Here's how the part is built. I have some questions about the finished solid (model axes, mm). A direction names the side the tool comes from. Round coordinates to 2 decimals unless told otherwise and drop trailing zeros. Write each loop counter-clockwise with the first axis right and the second up, starting at its lowest first coordinate (ties: lowest second). Pieces come first, ordered by that corner, then holes. Notation, with made-up numbers: (19.5, -32) -> (77.5, -32) arc R17 ccw to (77.5, -13) -> close; hole circle Ø7 at (39.25, 54.5). An arc over 180 degrees is marked (long way). Put each result on its own line as item: value. Start each with the question number.
1. I need wall thicknesses on probe 1 along X at (y, z) = (6.75, 0.5); probe 2 along Z at (x, y) = (-24.5, -1.5); probe 3 along Y at (x, z) = (-43.5, 2). Which ranges of each line are inside material? Lowest first, please. Write a range as from..to.
2. For pin 1 (10 mm diameter, centred on y = -8, z = -5, fed in from -X); pin 2 (4.5 mm diameter, centred on y = -3, z = -0.5, fed in from +X); pin 3 (4 mm diameter, centred on x = 27.5, z = 42.5, fed in from +Y); pin 4 (3 mm diameter, centred on x = 0.5, y = -4.5, fed in from +Z), each with a flat end and sliding along its axis, tell me the tip position at first contact or that it passes through.
3. Suppose I cut it at C-C (z = 0). Count the separate pieces of the cut face and the enclosed holes in it, then the cut area to 3 significant figures.
4. We'd pull the mould along X, two halves only. Please class faces 4 (the face through (0.515, 6.479, -49.897)), 5 (the face through (29.846, 4.93, 31.091)), 6 (the face through (26, -3, -10)): +X half, -X half, draft (parallel to the pull), parting line (faces both ways), or undercut.
5. Suppose I cut it at A-A (y = -2). Please give me the cut outline in (x, z).
6. Suppose I cut it at B-B (y = -10). Please give me the cut outline in (x, z), then the cut area to 3 significant figures.
7. Which directions (+Z, -Z, +X, -X, +Y, -Y) give clear straight access to the entire face, cutting with the end or side of a thin tool? Please do faces 1 (the face through (0, -5, 15)), 2 (the face through (21.71, -0.99, -2.53)), 3 (the face through (-28, 3.5, 3.2)).
```python
from build123d import *
from OCP.BRepFilletAPI import BRepFilletAPI_MakeChamfer

# Parameters (mm, degrees)
SKETCH_1_R          = 55
EXTRUDE_1_DEPTH     = 5
SKETCH_2_R          = 49.9
EXTRUDE_2_DEPTH     = 5
SKETCH_3_W          = 35
SKETCH_3_H          = 30
EXTRUDE_3_DEPTH     = 25
SKETCH_4_W          = 20.2
SKETCH_4_H          = 10.3
CUT_EXTRUDE_1_DEPTH = 93.466210045
SKETCH_5_R          = 4.1
CUT_EXTRUDE_2_DEPTH = 82.700673192
SKETCH_6_R          = 2.75
CUT_EXTRUDE_3_DEPTH = 86.293610546
CHAMFER1_SIZE       = 2
CHAMFER1_SIZE2      = 0.535898385
SKETCH2_W           = 35
SKETCH2_H           = 30
CUT_EXTRUDE1_DEPTH  = 12.5
BOSS_EXTRUDE1_START = -2
SKETCH4_W           = 70
SKETCH4_H           = 20
BOSS_EXTRUDE1_DEPTH = 5.35
SKETCH5_R           = 4.15
CUT_EXTRUDE2_DEPTH  = 80.281917882
CUT_EXTRUDE3_DEPTH  = 6.5
SKETCH7_W           = 20
SKETCH7_H           = 34
CUT_EXTRUDE4_DEPTH  = 5
CHAMFER2_SIZE       = 1
CHAMFER2_SIZE2      = 2.747477419


with BuildPart() as part:
    # Эскиз1 → Бобышка-Вытянуть1 (new body)
    with BuildSketch(Plane(origin=(0, 0, 0), x_dir=(1, 0, 0), z_dir=(0, 1, 0))):
        with Locations(Location((0, 0, 0), (0, 0, 270))):
            Circle(SKETCH_1_R)
    extrude(amount=EXTRUDE_1_DEPTH)

    # Эскиз2 → Бобышка-Вытянуть2 (add)
    with BuildSketch(Plane(origin=(0, 5, 0), x_dir=(1, 0, 0), z_dir=(0, 1, 0))):
        with Locations(Location((0, 0, 0), (0, 0, 270))):
            Circle(SKETCH_2_R)
    extrude(amount=EXTRUDE_2_DEPTH)

    # Эскиз3 → Бобышка-Вытянуть3 (add)
    with BuildSketch(Plane.XZ):
        Rectangle(SKETCH_3_W, SKETCH_3_H)
    extrude(amount=EXTRUDE_3_DEPTH)

    # Эскиз4 → Вырез-Вытянуть1 (cut, through all)
    with BuildSketch(Plane.XY.offset(15)):
        with Locations((0, -12.5)):
            Rectangle(SKETCH_4_W, SKETCH_4_H)
    extrude(amount=-CUT_EXTRUDE_1_DEPTH, mode=Mode.SUBTRACT)

    # Эскиз5 → Вырез-Вытянуть2 (cut, through all)
    with BuildSketch(Plane.XZ):
        with Locations(Location((33.592198598, -32.871936263, 0), (0, 0, 270))):
            Circle(SKETCH_5_R)
        with Locations(Location((-33.591727056, -32.872418125, 0), (0, 0, 270))):
            Circle(SKETCH_5_R)
        with Locations(Location((-33.591727056, 32.872418125, 0), (0, 0, 270))):
            Circle(SKETCH_5_R)
        with Locations(Location((33.483215177, 32.983215177, 0), (0, 0, 270))):
            Circle(SKETCH_5_R)
    extrude(amount=-CUT_EXTRUDE_2_DEPTH, mode=Mode.SUBTRACT)

    # Эскиз6 → Вырез-Вытянуть3 (cut, through all)
    with BuildSketch(Plane(origin=(0, 10, 0), x_dir=(1, 0, 0), z_dir=(0, 1, 0))):
        with Locations(Location((-17.999856554, 19.999999999, 0), (0, 0, 270))):
            Circle(SKETCH_6_R)
    extrude(amount=-CUT_EXTRUDE_3_DEPTH, mode=Mode.SUBTRACT)

    # Chamfer1: one chamfer whose edges measure the first distance from different faces: ONE call of the kernel's chamfer builder (chamfer() names one face for all edges)
    chamfer1_edges_1 = [part.edges().sort_by_distance(p)[0] for p in [
        (0.000357897, 10, -49.899999999),
    ]]
    chamfer1_side_1 = [part.faces().sort_by_distance(p)[0] for p in [
        (0.000357897, 7.5, -49.899999999),
    ]]
    chamfer1_edges_2 = [part.edges().sort_by_distance(p)[0] for p in [
        (-49.9, 10, 0),
    ]]
    chamfer1_side_2 = [part.faces().sort_by_distance(p)[0] for p in [
        (-49.9, 7.5, 0),
    ]]
    chamfer1_edges_3 = [part.edges().sort_by_distance(p)[0] for p in [
        (-0.08242255, 10, 49.899931929),
    ]]
    chamfer1_side_3 = [part.faces().sort_by_distance(p)[0] for p in [
        (-0.08242255, 7.5, 49.899931929),
    ]]
    chamfer1_edges_4 = [part.edges().sort_by_distance(p)[0] for p in [
        (49.899931657, 10, 0.082587101),
    ]]
    chamfer1_side_4 = [part.faces().sort_by_distance(p)[0] for p in [
        (49.899931657, 7.5, 0.082587101),
    ]]
    chamfer1 = BRepFilletAPI_MakeChamfer(part.part.solid().wrapped)
    for e in chamfer1_edges_1:
        chamfer1.Add(CHAMFER1_SIZE, CHAMFER1_SIZE2, e.wrapped, chamfer1_side_1[0].wrapped)  # the first distance lies on this face
    for e in chamfer1_edges_2:
        chamfer1.Add(CHAMFER1_SIZE, CHAMFER1_SIZE2, e.wrapped, chamfer1_side_2[0].wrapped)  # the first distance lies on this face
    for e in chamfer1_edges_3:
        chamfer1.Add(CHAMFER1_SIZE, CHAMFER1_SIZE2, e.wrapped, chamfer1_side_3[0].wrapped)  # the first distance lies on this face
    for e in chamfer1_edges_4:
        chamfer1.Add(CHAMFER1_SIZE, CHAMFER1_SIZE2, e.wrapped, chamfer1_side_4[0].wrapped)  # the first distance lies on this face
    add(Compound.cast(chamfer1.Shape()), mode=Mode.REPLACE)

    # Sketch2 → Cut-Extrude1 (cut)
    with BuildSketch(Plane.XZ.offset(25)):
        Rectangle(SKETCH2_W, SKETCH2_H)
    extrude(amount=-CUT_EXTRUDE1_DEPTH, mode=Mode.SUBTRACT)

    # Sketch4 → Boss-Extrude1 (add)
    with BuildSketch(Plane.XZ.offset(7.35).offset(BOSS_EXTRUDE1_START)):
        Rectangle(SKETCH4_W, SKETCH4_H)
    extrude(amount=-BOSS_EXTRUDE1_DEPTH)

    # Sketch5 → Cut-Extrude2 (cut, through all)
    with BuildSketch(Plane.XZ.offset(5.35)):
        with Locations((25, 0)):
            Circle(SKETCH5_R)
        with Locations((-25, 0)):
            Circle(SKETCH5_R)
    extrude(amount=-CUT_EXTRUDE2_DEPTH, mode=Mode.SUBTRACT)

    # Sketch6 → Cut-Extrude3 (cut)
    with BuildSketch(Plane(origin=(0, 10, 0), x_dir=(1, 0, 0), z_dir=(0, 1, 0))):
        Polygon((-18.504809472, 3.75), (-25, 7.5), (-31.495190528, 3.75), (-31.495190528, -3.75), (-25, -7.5), (-18.504809472, -3.75), align=None)
        Polygon((31.495190528, 3.75), (25, 7.5), (18.504809472, 3.75), (18.504809472, -3.75), (25, -7.5), (31.495190528, -3.75), align=None)
    extrude(amount=-CUT_EXTRUDE3_DEPTH, mode=Mode.SUBTRACT)

    # Sketch7 → Cut-Extrude4 (cut)
    with BuildSketch(Plane(origin=(0, 10, 0), x_dir=(1, 0, 0), z_dir=(0, 1, 0))):
        Rectangle(SKETCH7_W, SKETCH7_H)
    extrude(amount=-CUT_EXTRUDE4_DEPTH, mode=Mode.SUBTRACT)

    # Chamfer2
    chamfer2_edges = [part.edges().sort_by_distance(p)[0] for p in [
        (-18.504809472, 10, 0),
        (-21.752404736, 10, -5.625),
        (-28.247595264, 10, -5.625),
        (-31.495190528, 10, 0),
        (-28.247595264, 10, 5.625),
        (-21.752404736, 10, 5.625),
        (31.495190528, 10, 0),
        (28.247595264, 10, -5.625),
        (21.752404736, 10, -5.625),
        (18.504809472, 10, 0),
        (21.752404736, 10, 5.625),
        (28.247595264, 10, 5.625),
    ]]
    chamfer2_side = [part.faces().sort_by_distance(p)[0] for p in [
        (-28.121658773, 10, 32.336814493),
    ]]
    chamfer(chamfer2_edges, length=CHAMFER2_SIZE, length2=CHAMFER2_SIZE2, reference=chamfer2_side[0])


solid = part.part
```
Verdict:
1. probe 1: x = -49.9..-31.5, -18.5..-10, 10..18.5, 31.5..49.9
1. probe 2: z = -10..-4.12, 4.12..10
1. probe 3: y = 0..10
2. pin 1: stops at x = -35
2. pin 2: stops at x = 35
2. pin 3: stops at y = 10
2. pin 4: stops at z = 15
3. separate pieces: 3
3. enclosed holes: 0
3. area: 1,150 mm^2
4. face 4: parting line
4. face 5: undercut
4. face 6: draft
5. outline: (-35, -10) -> (-17.5, -10) -> (-17.5, -15) -> (17.5, -15) -> (17.5, -10) -> (35, -10) -> (35, 10) -> (17.5, 10) -> (17.5, 15) -> (-17.5, 15) -> (-17.5, 10) -> (-35, 10) -> close; hole circle Ø8.3 at (-25, 0); hole circle Ø8.3 at (25, 0)
6. outline: (-17.5, -15) -> (-10.1, -15) -> (-10.1, 15) -> (-17.5, 15) -> close; (10.1, -15) -> (17.5, -15) -> (17.5, 15) -> (10.1, 15) -> close
6. area: 444 mm^2
7. face 1: +Z, +X, -X, -Y
7. face 2: +Y, -Y
7. face 3: +Y
